Geometry check sheet. Reference: the model listing, model coordinates, mm. A direction names the side the tool comes from. Round coordinates to 2 decimals unless told otherwise and drop trailing zeros. Order: outer loops, then holes, each group sorted by start corner. A loop starts at its lowest first (then second) coordinate and runs counter-clockwise, first axis right, second up. Notation, with made-up numbers: (-30.75, -1.75) - (-23.75, -1.75) arc R17 cw to (-23.75, 24.25) - close; hole circle Ø5 at (60, 30.25). An arc over 180 degrees is marked (long way). Write each question's results on one line, items separated by ' | '.
```python
from build123d import *

# Parameters (mm, degrees)
F0_R     = 25
F1_DEPTH = 10
F2_R     = 24
F3_DEPTH = 6
F5_DEPTH = 6
F7_DEPTH = 6
F9_DEPTH = 6
F10_R    = 5


with BuildPart() as f1:
    # F0 (on Top) → F1 (new body)
    with BuildSketch(Plane.XY):
        Circle(F0_R)
    extrude(amount=F1_DEPTH)

    # F2 (on face) → F3 (cut)
    with BuildSketch(Plane.XY.offset(10)):
        Circle(F2_R)
    extrude(amount=-F3_DEPTH, mode=Mode.SUBTRACT)

    # F4 (on face) → F5 (join)
    with BuildSketch(Plane.XY.offset(4)):
        Polygon((2, 1.154701), (-2, 1.154701), (0, -2.309401), align=None)
    extrude(amount=F5_DEPTH)

    # F6 (on face) → F7 (join)
    with BuildSketch(Plane.XY.offset(4)):
        Polygon((0, 19.000366), (2.05507, 19.894137), (0, 20.787908), (-2.05507, 19.894137), align=None)
        Polygon((16.4548, 9.500183), (18.256363, 8.167325), (18.002856, 10.393954), (16.201293, 11.726812), align=None)
        Polygon((16.4548, -9.500183), (16.201293, -11.726812), (18.002856, -10.393954), (18.256363, -8.167325), align=None)
        Polygon((0, -19.000366), (-2.05507, -19.894137), (0, -20.787908), (2.05507, -19.894137), align=None)
        Polygon((-16.4548, -9.500183), (-18.256363, -8.167325), (-18.002856, -10.393954), (-16.201293, -11.726812), align=None)
        Polygon((-16.4548, 9.500183), (-16.201293, 11.726812), (-18.002856, 10.393954), (-18.256363, 8.167325), align=None)
    extrude(amount=F7_DEPTH)

    # F8 (on face) → F9 (join)
    with BuildSketch(Plane.XY.offset(4)):
        Polygon((0, -13.794267), (1.842263, -12.518255), (0, -11.294267), (-1.860011, -12.544267), align=None)
        Polygon((0, -7.016653), (1.842263, -5.792665), (0, -4.516653), (-1.877231, -5.792665), align=None)
        Polygon((6.0766, -3.508326), (5.937727, -1.300886), (3.911536, -2.258326), (4.07798, -4.522062), align=None)
        Polygon((11.946186, -6.897134), (11.762258, -4.663681), (9.781122, -5.647134), (9.933649, -7.88295), align=None)
        Polygon((6.0766, 3.508326), (4.095464, 4.491779), (3.911536, 2.258326), (5.955211, 1.270603), align=None)
        Polygon((1.877231, 5.792665), (0, 7.016653), (-1.842263, 5.792665), (0, 4.516653), align=None)
        Polygon((-6.0766, 3.508326), (-5.937727, 1.300886), (-3.911536, 2.258326), (-4.07798, 4.522062), align=None)
        Polygon((-6.0766, -3.508326), (-4.095464, -4.491779), (-3.911536, -2.258326), (-5.955211, -1.270603), align=None)
        Polygon((-11.946186, -6.897134), (-9.919995, -7.854574), (-9.781122, -5.647134), (-11.79366, -4.661317), align=None)
        Polygon((-11.946186, 6.897134), (-11.762258, 4.663681), (-9.781122, 5.647134), (-9.933649, 7.88295), align=None)
        Polygon((0, 11.294267), (1.860011, 12.544267), (0, 13.794267), (-1.842263, 12.518255), align=None)
        Polygon((11.946186, 6.897134), (9.919995, 7.854574), (9.781122, 5.647134), (11.79366, 4.661317), align=None)
    extrude(amount=F9_DEPTH)

    # F10
    f10_edges = [f1.edges().sort_by_distance(p)[0] for p in [
        (-25, 0, 0),
    ]]
    fillet(f10_edges, radius=F10_R)


solid = f1.part
```
(1) Material ranges on line 1 (X direction, y = -2.5, z = 4.5); line 2 (X direction, y = 3.5, z = 7); line 3 (Z direction, x = 3, y = -9), recorded low to high.
Answers follow:
line 1: -24.85 to -23.87, -6.02 to -3.93, 3.93 to 6.01, 23.87 to 24.85 | line 2: -24.75 to -23.74, -6.08 to -4, 4.01 to 6.08, 23.74 to 24.75 | line 3: 0 to 4
(2) Section check A-A (y = 0). Record the cut outline in (x, z).
Answers follow:
outline: (-25, 5) arc R5 ccw to (-20, 0) - (20, 0) arc R5 ccw to (25, 5) - (25, 10) - (24, 10) - (24, 4) - (1.33, 4) - (1.33, 10) - (-1.33, 10) - (-1.33, 4) - (-24, 4) - (-24, 10) - (-25, 10) - close
(3) Access from +Z, -Z, +X, -X, +Y, -Y to the whole of each face (thin tool, end or side, straight path). Record for faces 1 (the face through (5.1, 3.993, 6.958)), 2 (the face through (-5, 3, 10)).
Answers follow:
face 1: +Z | face 2: +Z, +X, -X, +Y, -Y
(4) Section check B-B (z = 1.25). Record the cut outline in (x, y).
Answers follow:
outline: circle Ø46.61 at (0, 0)
(5) Draft check along X on faces 3 (the face through (-1.042, -20.335, 6.958)), 4 (the face through (0, -20, 10)). Enter one of: released by +X, released by -X, zero draft, split by the parting line, or undercut.
Answers follow:
face 3: undercut | face 4: zero draft
(6) Depth check by flat-ended pin: pin 1 Ø6 at (y, z) = (-14, 1) entering from +X; pin 2 Ø4 at (x, z) = (-7.5, 5.5) entering from -Y; pin 3 Ø4.5 at (x, z) = (0.5, 8) entering from +Y. Enter the tip coordinate at first touch or a pass-through.
Answers follow:
pin 1: x = 21.59 | pin 2: y = -24.39 | pin 3: y = 25
